```python
from build123d import *

# Parameters (mm, degrees)
FORMSENKUNG_F_R_M5_LINSENSENKSCHRAUBE_MI_D           = 5.5
FORMSENKUNG_F_R_M5_LINSENSENKSCHRAUBE_MI_CSINK_D     = 10.4
FORMSENKUNG_F_R_M5_LINSENSENKSCHRAUBE_MI_CSINK_ANGLE = 90
SKIZZE7_W                                            = 1
SKIZZE7_H                                            = 6
SCHNITT_LINEAR_AUSTRAGEN1_DEPTH                      = 66.531976927


with BuildPart() as part:
    # Skizze2 → Rotation1 (revolve)
    with BuildSketch(Plane(origin=(0, 0, 0), x_dir=(1, 0, 0), z_dir=(0, 1, 0))):
        Polygon((48, -35), (52, -35), (52, -29), (52, -28), (48, -28), (48, -29), align=None)
    revolve(axis=Axis((52, 0, 29), (0, 0, 1)))

    # Formsenkung für M5 Linsensenkschraube mit Schlitz1 (through all)
    with Locations(Plane.XY.offset(35)):
        with Locations((52, 0)):
            CounterSinkHole(FORMSENKUNG_F_R_M5_LINSENSENKSCHRAUBE_MI_D / 2, FORMSENKUNG_F_R_M5_LINSENSENKSCHRAUBE_MI_CSINK_D / 2, counter_sink_angle=FORMSENKUNG_F_R_M5_LINSENSENKSCHRAUBE_MI_CSINK_ANGLE)

    # Skizze7 → Schnitt-Linear austragen1 (cut, symmetric)
    with BuildSketch(Plane(origin=(0, 0, 0), x_dir=(1, 0, 0), z_dir=(0, 1, 0))):
        with Locations((51.5, -32)):
            Rectangle(SKIZZE7_W, SKIZZE7_H)
    schnitt_linear_austragen1 = extrude(amount=SCHNITT_LINEAR_AUSTRAGEN1_DEPTH, both=True, mode=Mode.SUBTRACT)

    # Spiegeln1: Schnitt-Linear austragen1 across plane
    add(schnitt_linear_austragen1.mirror(Plane(origin=(52, -4, 29), x_dir=(0, 0, 1), z_dir=(1, 0, 0))), mode=Mode.SUBTRACT)


solid = part.part
```
Input: part model. Units: mm. Frame: model coordinates. A direction names the side the tool comes from. Round coordinates to 2 decimals unless told otherwise and drop trailing zeros. Loops run counter-clockwise (first coordinate to the right, second up) from the corner with the lowest first, then second, coordinate; pieces in that order, holes last. Notation, with made-up numbers: (37, 33) -> (52, 33) arc R22 ccw to (52, 70) -> close; hole circle Ø7 at (76, -5). An arc over 180 degrees is marked (long way). Write each question's results on one line, items separated by ' | '.
1. Set-up query: faces 4 (the face through (49.46, -1.05, 30.24)), 5 (the face through (49.1, -0.1, 32.7)), 6 (the face through (53, -3, 31)). Return all of +Z, -Z, +X, -X, +Y, -Y with unobstructed straight access to the full face (end or side cutting, diameter ignored); none if empty.
Geometry results:
face 4: +Z, -Z | face 5: +Z | face 6: +Z, +Y, -Y
2. Mould query, pull axis X, two halves, no side actions, for faces 1 (the face through (55, -1, 28)), 2 (the face through (54.9, 0.1, 32.7)), 3 (the face through (48.185, -1.201, 30.941)). Classes: +X half, -X half, draft (parallel to the pull), parting line (faces both ways), or undercut.
Geometry results:
face 1: draft | face 2: undercut | face 3: parting line
3. Section A-A (x = 52). Return loops of the section in (y, z).
Geometry results:
outline: (-4, 28) -> (-2.75, 28) -> (-2.75, 29) -> (-4, 29) -> close; (2.75, 28) -> (4, 28) -> (4, 29) -> (2.75, 29) -> close
4. Ray query, line 1 (Y direction, x = 52, z = 28.95); line 2 (X direction, y = 0, z = 31.3); line 3 (Y direction, x = 53.75, z = 29.2). Return the intervals inside material, ascending. Write a range as from..to.
Geometry results:
line 1: -4..-2.75, 2.75..4 | line 2: 48..49.25, 54.75..56 | line 3: -3.6..-2.12, 2.12..3.6
5. First-contact query: P1, Ø0.7, axis at y = -3.5, z = 30.5, coming from the -X side; P2, Ø1.4, axis at y = 3.5, z = 31, coming from the +X side. Flat tips, straight axial feed; report the tip coordinate or a pass-through.
Geometry results:
P1: x = 49.53 | P2: x = 54.86
6. Section B-B (y = 0). Return loops of the section in (x, z), and give its area (3 significant figures).
Geometry results:
outline: (48, 28) -> (49.25, 28) -> (49.25, 32.55) -> (48, 33.8) -> close; (54.75, 28) -> (56, 28) -> (56, 33.8) -> (54.75, 32.55) -> close | area: 12.9 mm2
